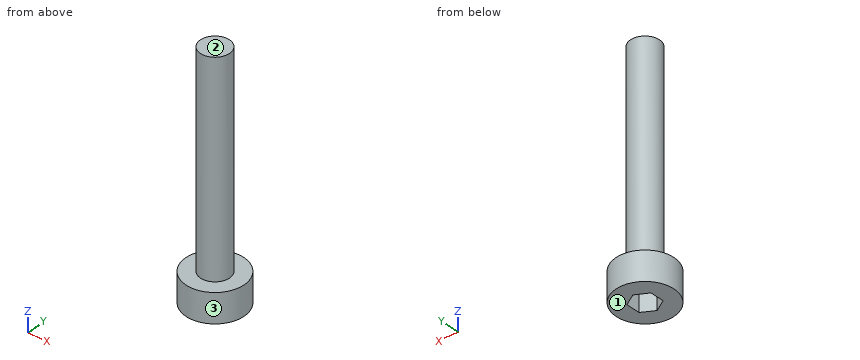
```python
from build123d import *

# Parameters (mm, degrees)
SKETCH_1_R          = 1.4
EXTRUDE_1_DEPTH     = 1.4
SKETCH_2_R          = 0.7
EXTRUDE_2_DEPTH     = 10
CUT_EXTRUDE_1_DEPTH = 1


with BuildPart() as part:
    # 草图1 → 凸台-拉伸1 (new body)
    with BuildSketch(Plane.XY):
        Circle(SKETCH_1_R)
    extrude(amount=EXTRUDE_1_DEPTH)

    # 草图2 → 凸台-拉伸2 (add)
    with BuildSketch(Plane.XY.offset(1.4)):
        Circle(SKETCH_2_R)
    extrude(amount=EXTRUDE_2_DEPTH)

    # 草图3 → 切除-拉伸1 (cut)
    with BuildSketch(Plane(origin=(0, 0, 0), x_dir=(-1, 0, 0), z_dir=(0, 0, -1))):
        Polygon((0, 0.68), (-0.588897275, 0.34), (-0.588897275, -0.34), (0, -0.68), (0.588897275, -0.34), (0.588897275, 0.34), align=None)
    extrude(amount=-CUT_EXTRUDE_1_DEPTH, mode=Mode.SUBTRACT)


solid = part.part
```
CAD build for the part. Positions are in the model's coordinates, mm. Face numbers are marked on the shaded views. Give positions to 0.01 mm unless a question says otherwise; leave off trailing zeros. Write each loop counter-clockwise with the first axis right and the second up, starting at its lowest first coordinate (ties: lowest second). Pieces come first, ordered by that corner, then holes. Notation, with made-up numbers: M 43,5.25 L 87,5.25 A33 cw 87,42.25 Z; hole C -24.75,-0.75 d4. An arc over 180 degrees is marked long. Return JSON: item names as keys, results as strings. Group by question number.
(1) Band-saw the part on B-B (x = -0.3). Give the cut face in (y, z), and give its area (3 significant figures).
(2) Band-saw the part on A-A (y = 0). Give the cut face in (x, z).
(3) Band-saw the part on C-C (x = 1.05). Give the cut face in (y, z), and give its area (3 significant figures).
(4) Drill centre lines: L1, parallel to Z at x = 0.8, y = -0.65; L2, parallel to Z at x = 0, y = -0.35; L3, parallel to X at y = -0.3, z = 3. Where is each one in solid material? Low to high. Write a range as [from, to].
(5) Mould opens along Z. For the marked faces 1, 2 and 3 say: pulls with the +Z half, pulls with the -Z half, needs draft (parallel to the pull), parting line crosses it, or undercut.
(6) Flat gauge pins, fed straight in: pin 1 Ø1 at (y, z) = (-0.5, 4) entering from +X; pin 2 Ø0.6 at (x, y) = (0, 0) entering from -Z. Where does each tip first touch, or does it go through?
(7) Band-saw the part on D-D (y = -1.1). Give the cut face in (x, z).
Entries:
{
 "1": {"outline": "M -1.37,0 L -0.51,0 L -0.51,1 L 0.51,1 L 0.51,0 L 1.37,0 L 1.37,1.4 L 0.63,1.4 L 0.63,11.4 L -0.63,11.4 L -0.63,1.4 L -1.37,1.4 Z", "area": "15.5 mm^2"},
 "2": {"outline": "M -1.4,0 L -0.59,0 L -0.59,1 L 0.59,1 L 0.59,0 L 1.4,0 L 1.4,1.4 L 0.7,1.4 L 0.7,11.4 L -0.7,11.4 L -0.7,1.4 L -1.4,1.4 Z"},
 "3": {"outline": "M -0.93,0 L 0.93,0 L 0.93,1.4 L -0.93,1.4 Z", "area": "2.59 mm^2"},
 "4": {"L1": "z = [0, 1.4]", "L2": "z = [1, 11.4]", "L3": "x = [-0.63, 0.63]"},
 "5": {"face 1": "pulls with the -Z half", "face 2": "pulls with the +Z half", "face 3": "needs draft"},
 "6": {"pin 1": "stops at x = 0.7", "pin 2": "stops at z = 1"},
 "7": {"outline": "M -0.87,0 L 0.87,0 L 0.87,1.4 L -0.87,1.4 Z"}
}
